```python
from build123d import *

# Parameters (mm, degrees)
SKETCH1_W           = 95
SKETCH1_H           = 50.55
SKETCH1_R           = 1.75
SKETCH1_R_2         = 3.75
SKETCH1_R_3         = 4.3
BOSS_EXTRUDE1_DEPTH = 1.5
CUT_EXTRUDE1_DEPTH  = 1.5
FILLET1_R           = 3
SKETCH3_R           = 4.9
SKETCH3_R_2         = 4.3
BOSS_EXTRUDE2_DEPTH = 1.5
SKETCH5_W           = 6.5
SKETCH5_H           = 4
BOSS_EXTRUDE3_DEPTH = 4.4
CUT_EXTRUDE2_REACH  = 56.128
SKETCH6_R           = 1.25
SKETCH8_R           = 2.05
CUT_EXTRUDE3_DEPTH  = 1.5
FILLET2_R           = 2.25


with BuildPart() as part:
    # Sketch1 → Boss-Extrude1 (new body)
    with BuildSketch(Plane(origin=(0, 0, 0), x_dir=(1, 0, 0), z_dir=(0, 1, 0))):
        Rectangle(SKETCH1_W, SKETCH1_H)
        with Locations(Location((-42.5, 20.275, 0), (0, 0, 270))):
            Circle(SKETCH1_R, mode=Mode.SUBTRACT)
        with Locations(Location((42.5, 20.275, 0), (0, 0, 90))):
            Circle(SKETCH1_R, mode=Mode.SUBTRACT)
        with Locations(Location((42.5, -20.275, 0), (0, 0, 270))):
            Circle(SKETCH1_R, mode=Mode.SUBTRACT)
        with Locations(Location((-42.5, -20.275, 0), (0, 0, 90))):
            Circle(SKETCH1_R, mode=Mode.SUBTRACT)
        with Locations(Location((-13.1, 0, 0), (0, 0, 270))):
            Circle(SKETCH1_R_2, mode=Mode.SUBTRACT)
        with Locations(Location((13.1, 0, 0), (0, 0, 90))):
            Circle(SKETCH1_R_2, mode=Mode.SUBTRACT)
        with Locations(Location((0, 13.1, 0), (0, 0, 270))):
            Circle(SKETCH1_R_2, mode=Mode.SUBTRACT)
        with Locations(Location((0, -13.1, 0), (0, 0, 90))):
            Circle(SKETCH1_R_2, mode=Mode.SUBTRACT)
        with Locations(Location((-41.2, 0, 0), (0, 0, 270))):
            Circle(SKETCH1_R_3, mode=Mode.SUBTRACT)
    extrude(amount=BOSS_EXTRUDE1_DEPTH)

    # Sketch2 → Cut-Extrude1 (cut)
    with BuildSketch(Plane(origin=(0, 1.5, 0), x_dir=(1, 0, 0), z_dir=(0, 1, 0))):
        Polygon((-32.5, 20.275), (32.5, 20.275), (37.5, 25.275), (-37.5, 25.275), align=None)
        Polygon((37.5, -25.275), (32.5, -20.275), (-32.5, -20.275), (-37.5, -25.275), align=None)
        Polygon((47.5, -15.275), (47.5, 15.275), (42.5, 10.275), (42.5, -10.275), align=None)
    extrude(amount=-CUT_EXTRUDE1_DEPTH, mode=Mode.SUBTRACT)

    # Fillet1
    fillet1_edges = [part.edges().sort_by_distance(p)[0] for p in [
        (37.5, 0.75, -25.275),
        (32.5, 0.75, -20.275),
        (-32.5, 0.75, -20.275),
        (-37.5, 0.75, -25.275),
        (-37.5, 0.75, 25.275),
        (-32.5, 0.75, 20.275),
        (32.5, 0.75, 20.275),
        (37.5, 0.75, 25.275),
        (47.5, 0.75, 25.275),
        (-47.5, 0.75, 25.275),
        (-47.5, 0.75, -25.275),
        (47.5, 0.75, -25.275),
        (47.5, 0.75, 15.275),
        (42.5, 0.75, 10.275),
        (42.5, 0.75, -10.275),
        (47.5, 0.75, -15.275),
    ]]
    fillet(fillet1_edges, radius=FILLET1_R)

    # Sketch3 → Boss-Extrude2 (add)
    with BuildSketch(Plane(origin=(0, 1.5, 0), x_dir=(1, 0, 0), z_dir=(0, 1, 0))):
        with Locations(Location((-41.2, 0, 0), (0, 0, 270))):
            Circle(SKETCH3_R)
        with Locations(Location((-41.2, 0, 0), (0, 0, 270))):
            Circle(SKETCH3_R_2, mode=Mode.SUBTRACT)
    extrude(amount=BOSS_EXTRUDE2_DEPTH)

    # Sketch5 → Boss-Extrude3 (add)
    with BuildSketch(Plane(origin=(0, 1.5, 0), x_dir=(1, 0, 0), z_dir=(0, 1, 0))):
        with Locations((-44.25, -7.025)):
            Rectangle(SKETCH5_W, SKETCH5_H)
        with Locations((-44.25, -15.525)):
            Rectangle(SKETCH5_W, SKETCH5_H)
    extrude(amount=BOSS_EXTRUDE3_DEPTH)

    # Sketch6 → Cut-Extrude2 (cut, up to next)
    with BuildSketch(Plane(origin=(0, 5.9, 0), x_dir=(1, 0, 0), z_dir=(0, 1, 0)), mode=Mode.PRIVATE) as cut_extrude2_sk1:
        with Locations(Location((-44.25, -7.025, 0), (0, 0, 270))):
            Circle(SKETCH6_R)
    cut_extrude2_tool1 = extrude(cut_extrude2_sk1.sketch, amount=-CUT_EXTRUDE2_REACH, mode=Mode.PRIVATE) & part.part
    # Sketch6 → Cut-Extrude2 (cut, up to next)
    with BuildSketch(Plane(origin=(0, 5.9, 0), x_dir=(1, 0, 0), z_dir=(0, 1, 0)), mode=Mode.PRIVATE) as cut_extrude2_sk2:
        with Locations(Location((-44.25, -15.525, 0), (0, 0, 270))):
            Circle(SKETCH6_R)
    cut_extrude2_tool2 = extrude(cut_extrude2_sk2.sketch, amount=-CUT_EXTRUDE2_REACH, mode=Mode.PRIVATE) & part.part
    add(cut_extrude2_tool1.solids().sort_by_distance((-44.25, 5.9, 7.025))[0], mode=Mode.SUBTRACT)
    add(cut_extrude2_tool2.solids().sort_by_distance((-44.25, 5.9, 15.525))[0], mode=Mode.SUBTRACT)

    # Sketch8 → Cut-Extrude3 (cut)
    with BuildSketch(Plane.XZ):
        with Locations(Location((-44.25, 15.525, 0), (0, 0, 270))):
            Circle(SKETCH8_R)
        with Locations(Location((-44.25, 7.025, 0), (0, 0, 270))):
            Circle(SKETCH8_R)
    extrude(amount=-CUT_EXTRUDE3_DEPTH, mode=Mode.SUBTRACT)

    # Fillet2
    # the kernel refuses this fillet: 2.25 mm, written as the material it adds along each edge
    with BuildSketch(Plane(origin=(-39.075, 1.5, 13.525), x_dir=(0, 0, -1), z_dir=(-1, 0, 0))) as fillet2_piece_1_section:
        with BuildLine():
            CenterArc((FILLET2_R, -FILLET2_R), FILLET2_R, 90, 90)
            Line((0, -FILLET2_R), (0, 0))
            Line((0, 0), (FILLET2_R, 0))
        make_face()
    fillet2_piece_1 = extrude(amount=8.425, mode=Mode.PRIVATE)
    fillet2_piece_1 = fillet2_piece_1 - Plane(origin=(-44.25, 1.998463369, 15.525), x_dir=(0, 0, -1), z_dir=(0, -1, 0)) * Cylinder(2.05, 26, mode=Mode.PRIVATE)
    fillet2_piece_1 = split(fillet2_piece_1, bisect_by=Plane(origin=(-41, 1.998463369, 13.018330937), z_dir=(-1, 0, 0)), keep=Keep.TOP, mode=Mode.PRIVATE)
    add(fillet2_piece_1)
    with BuildSketch(Plane(origin=(-41, 1.5, 13.525), x_dir=(0, 0, -1), z_dir=(-1, 0, 0))) as fillet2_piece_2_section:
        with BuildLine():
            CenterArc((FILLET2_R, -FILLET2_R), FILLET2_R, 90, 90)
            Line((0, -FILLET2_R), (0, 0))
            Line((0, 0), (FILLET2_R, 0))
        make_face()
    fillet2_piece_2 = extrude(amount=8.425, mode=Mode.PRIVATE)
    fillet2_piece_2 = split(fillet2_piece_2, bisect_by=Plane(origin=(-47.5, 1.998463369, 13.018330937), z_dir=(1, 0, 0)), keep=Keep.TOP, mode=Mode.PRIVATE)
    fillet2_piece_2 = fillet2_piece_2 - Plane(origin=(-44.25, 1.998463369, 15.525), x_dir=(0, 0, -1), z_dir=(0, -1, 0)) * Cylinder(2.05, 26, mode=Mode.PRIVATE)
    add(fillet2_piece_2)
    with BuildSketch(Plane(origin=(-47.5, 1.5, 9.025), x_dir=(0, 0, 1), z_dir=(1, 0, 0))) as fillet2_piece_3_section:
        with BuildLine():
            CenterArc((FILLET2_R, -FILLET2_R), FILLET2_R, 90, 90)
            Line((0, -FILLET2_R), (0, 0))
            Line((0, 0), (FILLET2_R, 0))
        make_face()
    fillet2_piece_3 = extrude(amount=8.425, mode=Mode.PRIVATE)
    fillet2_piece_3 = fillet2_piece_3 - Plane(origin=(-44.25, 1.998463384, 7.025), x_dir=(0, 0, -1), z_dir=(0, -1, 0)) * Cylinder(2.05, 26, mode=Mode.PRIVATE)
    fillet2_piece_3 = split(fillet2_piece_3, bisect_by=Plane(origin=(-41, 1.998463384, 9.531669097), z_dir=(-1, 0, 0)), keep=Keep.TOP, mode=Mode.PRIVATE)
    add(fillet2_piece_3)
    with BuildSketch(Plane(origin=(-49.425, 1.5, 9.025), x_dir=(0, 0, 1), z_dir=(1, 0, 0))) as fillet2_piece_4_section:
        with BuildLine():
            CenterArc((FILLET2_R, -FILLET2_R), FILLET2_R, 90, 90)
            Line((0, -FILLET2_R), (0, 0))
            Line((0, 0), (FILLET2_R, 0))
        make_face()
    fillet2_piece_4 = extrude(amount=8.425, mode=Mode.PRIVATE)
    fillet2_piece_4 = split(fillet2_piece_4, bisect_by=Plane(origin=(-47.5, 1.998463384, 9.531669097), z_dir=(1, 0, 0)), keep=Keep.TOP, mode=Mode.PRIVATE)
    fillet2_piece_4 = fillet2_piece_4 - Plane(origin=(-44.25, 1.998463384, 7.025), x_dir=(0, 0, -1), z_dir=(0, -1, 0)) * Cylinder(2.05, 26, mode=Mode.PRIVATE)
    add(fillet2_piece_4)


solid = part.part
```
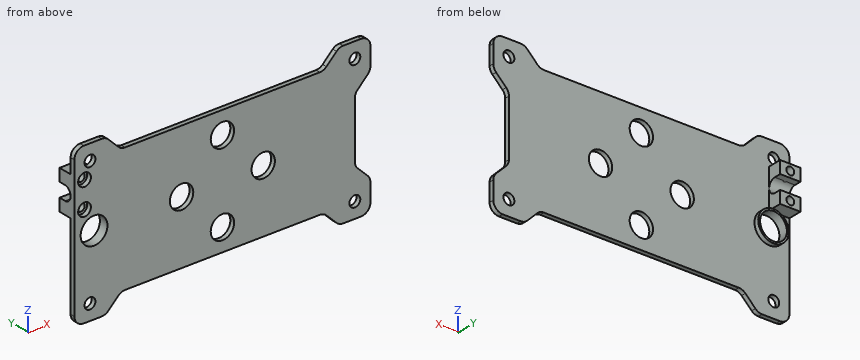
Geometry check sheet. Reference: the model listing, model coordinates, mm. Coordinates: 2 decimals unless noted, no trailing zeros. Order: outer loops, then holes, each group sorted by start corner. A loop starts at its lowest first (then second) coordinate and runs counter-clockwise, first axis right, second up.
Item 1: Section check B-B (x = 13.1). Enter the section's corners in (y, z) (3 decimals).
Item 2: Section check C-C (z = -13.5). Enter the section's corners in (x, y) (3 decimals).
Item 3: Section check D-D (x = -20). Enter the section's corners in (y, z) (3 decimals), plus the area to 3 significant figures.
Item 4: Depth check by flat-ended pin: pin 1 (2 mm diameter, centred on x = -43, y = 4.5, fed in from -Z) (3 decimals); pin 2 (1.2 mm diameter, centred on x = -45, z = 6, fed in from -Y); pin 3 (2 mm diameter, centred on x = -45, y = 3.5, fed in from +Z) (3 decimals). Enter the tip coordinate at first touch or a pass-through.
Item 5: Section check A-A (z = 0). Enter the section's corners in (x, y).
Item 6: Scan lines: line 1 along X through (y, z) = (0.75, 0); line 2 along X through (y, z) = (1.45, -1); line 3 along Z through (x, y) = (7.5, 0.65) (3 decimals). Record each from-to range of solid material in increasing order.
Check sheet entries:
1. outline: (0, -20.275) - (1.5, -20.275) - (1.5, -3.75) - (0, -3.75) - close; (0, 3.75) - (1.5, 3.75) - (1.5, 20.275) - (0, 20.275) - close
2. outline: (-47.5, 0) - (-3.729, 0) - (-3.729, 1.5) - (-47.5, 1.5) - close; (3.729, 0) - (45.725, 0) - (45.725, 1.5) - (3.729, 1.5) - close
3. outline: (0, -20.275) - (1.5, -20.275) - (1.5, 20.275) - (0, 20.275) - close
3. area: 60.8 mm2
4. pin 1: stops at z = 5.025
4. pin 2: stops at y = 1.5
4. pin 3: stops at z = 17.525
5. outline: (-47.5, 0) - (-45.5, 0) - (-45.5, 3) - (-46.1, 3) - (-46.1, 1.5) - (-47.5, 1.5) - close; (-36.9, 0) - (-16.85, 0) - (-16.85, 1.5) - (-36.3, 1.5) - (-36.3, 3) - (-36.9, 3) - close; (-9.35, 0) - (9.35, 0) - (9.35, 1.5) - (-9.35, 1.5) - close; (16.85, 0) - (42.5, 0) - (42.5, 1.5) - (16.85, 1.5) - close
6. line 1: x = -47.5 to -45.5, -36.9 to -16.85, -9.35 to 9.35, 16.85 to 42.5
6. line 2: x = -47.5 to -45.38, -37.02 to -16.71, -9.49 to 9.49, 16.71 to 42.5
6. line 3: z = -20.275 to 20.275
